Work out the finished part from the listing and answer in its coordinate system (mm). A direction names the side the tool comes from. Coordinates: 2 decimals unless noted, no trailing zeros. Loops run counter-clockwise (first coordinate to the right, second up) from the corner with the lowest first, then second, coordinate; pieces in that order, holes last.
```python
from build123d import *

# Parameters (mm, degrees)
F1_DEPTH = 15
F3_DEPTH = 46.3032221559
F5_D     = 4
F6_R     = 10
F7_SIZE  = 5


with BuildPart() as f1:
    # F0 (on Front) → F1 (new body, symmetric)
    with BuildSketch(Plane.XZ):
        Polygon((0, 8), (0, 0), (46.2695387348, 0), (78.4089192191, -38.3022221559), (82.1393804843, -30.3022221559), (50, 8), align=None)
    extrude(amount=F1_DEPTH, both=True)

    # F2 (on face) → F3 (cut, through all)
    with BuildSketch(Plane.XY.offset(8)):
        with BuildLine():
            ThreePointArc((15, 3), (12, 0), (15, -3))
            Line((15, -3), (35, -3))
            ThreePointArc((35, -3), (38, 0), (35, 3))
            Line((35, 3), (15, 3))
        make_face()
    extrude(amount=-F3_DEPTH, mode=Mode.SUBTRACT)

    # F5 (through all)
    with Locations(Plane(origin=(33.2804354537, 0, 27.9256011146), x_dir=(0, 1, 0), z_dir=(0.7660444431, 0, 0.6427876097))):
        with Locations((0, -41.0110249394), (0, -61.0110249394)):
            Hole(F5_D / 2)

    # F6
    f6_edges = [f1.edges().sort_by_distance(p)[0] for p in [
        (80.27415, -15, -34.302222),
        (80.27415, 15, -34.302222),
    ]]
    fillet(f6_edges, radius=F6_R)

    # F7
    f7_edges = [f1.edges().sort_by_distance(p)[0] for p in [
        (0, 15, 4),
        (0, -15, 4),
    ]]
    chamfer(f7_edges, length=F7_SIZE)


solid = f1.part
```
1. A cutting plane is placed at C-C, the plane y = 4. Give the vertices of the cut face in (x, z), then the cut area to 3 significant figures.
2. Straight lines are drawn through the part: probe 1 along Y at (x, z) = (17, 1); probe 2 along Z at (x, y) = (10.5, -1.5); probe 3 along X at (y, z) = (0, -6). For each, find the intervals that lie inside material, in ascending order.
3. A cutting plane is placed at A-A, the plane x = 31. Give the vertices of the cut face in (y, z), then the cut area to 3 significant figures.
4. A cutting plane is placed at B-B, the plane z = 1.5. Give the vertices of the cut face in (x, y).
5. Determine the mould class of faces 4 (the cylindrical face through (78.574, -12.148, -30.833)), 5 (the cylindrical face through (70.65, 0.43, -22.91)), 6 (the flat face through (62.11, -0.21, -18.88)) for opening direction X: released by +X, released by -X, zero draft, split by the parting line, or undercut.
6. A cutting plane is placed at D-D, the plane y = 0. Give the vertices of the cut face in (x, z).
7. Each of these flat-tipped pins is pushed along its axis until it touches: P1, Ø4, axis at y = -5.5, z = -0.5, coming from the +X side; P2, Ø1, axis at x = 57, y = 10.5, coming from the -Z side; P3, Ø1, axis at y = 1, z = -12.5, coming from the -X side. Where does it stop, or does it pass through?
8. For faces 1 (the flat face through (23, -4, 0)), 2 (the flat face through (42.5, -15, 0.4)), 3 (the cylindrical face through (12, 0, 4)), determine the directions among +Z, -Z, +X, -X, +Y, -Y from which every point of the face is accessible in a straight line to the end or side of a thin tool.
Answers below:
1. outline: (0, 0) - (46.27, 0) - (78.41, -38.3) - (82.14, -30.3) - (50, 8) - (0, 8) - close
1. area: 785 mm2
2. probe 1: y = -15 to -3, 3 to 15
2. probe 2: z = 0 to 8
2. probe 3: x = 51.3 to 53.54, 59.76 to 61.75
3. outline: (-15, 0) - (-3, 0) - (-3, 8) - (-15, 8) - close; (3, 0) - (15, 0) - (15, 8) - (3, 8) - close
3. area: 192 mm2
4. outline: (0, -10) - (5, -15) - (55.45, -15) - (55.45, 15) - (5, 15) - (0, 10) - close; hole (15, -3) - (35, -3) arc R3 ccw to (35, 3) - (15, 3) arc R3 ccw to start
5. face 4: released by +X
5. face 5: undercut
5. face 6: released by -X
6. outline: (0, 0) - (12, 0) - (12, 8) - (0, 8) - close; (38, 0) - (46.27, 0) - (52.23, -7.1) - (58.36, -1.96) - (50, 8) - (38, 8) - close; (54.8, -10.17) - (65.08, -22.42) - (71.21, -17.28) - (60.93, -5.02) - close; (67.65, -25.49) - (78.41, -38.3) - (82.14, -30.3) - (73.78, -20.34) - close
7. P1: stops at x = 58.81
7. P2: stops at z = -13.38
7. P3: stops at x = 56.34
8. face 1: -Z, -X, +Y, -Y
8. face 2: +Z, -Z, +X, -X, -Y
8. face 3: +Z, -Z
